Build history of the part. All positions in model axes, mm. A direction names the side the tool comes from. Give positions to 0.01 mm unless a question says otherwise; leave off trailing zeros. Order: outer loops, then holes, each group sorted by start corner. A loop starts at its lowest first (then second) coordinate and runs counter-clockwise, first axis right, second up. Notation, with made-up numbers: (-6, 5.25) - (30, 5.25) arc R24 ccw to (30, 24.25) - close; hole circle Ø8 at (39, -24). An arc over 180 degrees is marked (long way). One line per item, written item: value.
```python
from build123d import *

# Parameters (mm, degrees)
SKETCH_1_W          = 56
SKETCH_1_H          = 70
EXTRUDE_1_DEPTH     = 5
SKETCH_2_R          = 2
CUT_EXTRUDE_1_DEPTH = 5
SKETCH_5_W          = 25
SKETCH_5_H          = 28.7
EXTRUDE_3_DEPTH     = 4.5
SKETCH_6_W          = 32
SKETCH_6_H          = 40
EXTRUDE_4_DEPTH     = 15
SKETCH_9_R          = 2.15
CUT_EXTRUDE_2_DEPTH = 10
CUT_EXTRUDE_3_DEPTH = 10
CHAMFER_START       = -5
CHAMFER_1_DEPTH     = 40
CHAMFER_1_2_DEPTH   = 10
CHAMFER_START_2     = 25
CHAMFER_1_3_DEPTH   = 10
CHAMFER_START_3     = 5
CHAMFER_1_4_DEPTH   = 3
CHAMFER_2_SIZE      = 15
CHAMFER_3_SIZE      = 5


with BuildPart() as part:
    # 草图1 → 凸台-拉伸1 (new body)
    with BuildSketch(Plane.XY):
        Rectangle(SKETCH_1_W, SKETCH_1_H)
    extrude(amount=EXTRUDE_1_DEPTH)

    # 草图2 → 切除-拉伸1 (cut)
    with BuildSketch(Plane.XY.offset(5)):
        with Locations((-16, -28.4)):
            Circle(SKETCH_2_R)
        with Locations((-16, -14.4)):
            Circle(SKETCH_2_R)
    cut_extrude_1 = extrude(amount=-CUT_EXTRUDE_1_DEPTH, mode=Mode.SUBTRACT)

    # 镜向1: 切除-拉伸1 across plane
    add(cut_extrude_1.mirror(Plane(origin=(0, 0, 0), x_dir=(0, 0, 1), z_dir=(1, 0, 0))), mode=Mode.SUBTRACT)

    # 草图5 → 凸台-拉伸3 (add)
    with BuildSketch(Plane.XY.offset(5)):
        with Locations((15.5, 20.65)):
            Rectangle(SKETCH_5_W, SKETCH_5_H)
    extrude(amount=EXTRUDE_3_DEPTH)

    # 草图6 → 凸台-拉伸4 (add)
    with BuildSketch(Plane.ZY.offset(28)):
        with Locations((16, 15)):
            Rectangle(SKETCH_6_W, SKETCH_6_H)
    extrude(amount=EXTRUDE_4_DEPTH)

    # 草图9 → 切除-拉伸2 (cut)
    with BuildSketch(Plane.XY.offset(32)):
        with Locations((-35.5, 28)):
            Circle(SKETCH_9_R)
        with Locations(Location((-35.5, 2, 0), (0, 0, 180))):
            Circle(SKETCH_9_R)
    extrude(amount=-CUT_EXTRUDE_2_DEPTH, mode=Mode.SUBTRACT)

    # 草图10 → 切除-拉伸3 (cut)
    with BuildSketch(Plane.XY.offset(5)):
        with BuildLine():
            Line((-20, 5), (-20, 25))
            ThreePointArc((-20, 25), (-18, 27), (-16, 25))
            Line((-16, 25), (-16, 5))
            ThreePointArc((-16, 5), (-18, 3), (-20, 5))
        make_face()
    extrude(amount=-CUT_EXTRUDE_3_DEPTH, mode=Mode.SUBTRACT)

    # 倒角1: read off the stored shape, not the designer's step
    # 倒角1 outline → 倒角1 (add)
    with BuildSketch(Plane(origin=(0, 0, 0), x_dir=(1, 0, 0), z_dir=(0, 1, 0)).offset(CHAMFER_START)):
        Polygon((-20, -7), (-20, -5), (-28, -5), (-28, -15), align=None)
    extrude(amount=CHAMFER_1_DEPTH)

    # Chamfer 1 2 outline → Chamfer 1 2 (add)
    with BuildSketch(Plane(origin=(0, 0, 0), x_dir=(1, 0, 0), z_dir=(0, 1, 0)).offset(CHAMFER_START)):
        Polygon((-18, -5), (-20, -5), (-20, -7), align=None)
    extrude(amount=CHAMFER_1_2_DEPTH)

    # Chamfer 1 3 outline → Chamfer 1 3 (add)
    with BuildSketch(Plane(origin=(0, 0, 0), x_dir=(1, 0, 0), z_dir=(0, 1, 0)).offset(CHAMFER_START_2)):
        Polygon((-18, -5), (-20, -5), (-20, -7), align=None)
    extrude(amount=CHAMFER_1_3_DEPTH)

    # Chamfer 1 4 outline → Chamfer 1 4 (cut)
    with BuildSketch(Plane.XY.offset(CHAMFER_START_3)):
        with BuildLine():
            Line((-16, 5), (-20, 5))
            ThreePointArc((-20, 5), (-18, 3), (-16, 5))
        make_face()
        with BuildLine():
            Line((-20, 25), (-16, 25))
            ThreePointArc((-16, 25), (-18, 27), (-20, 25))
        make_face()
    extrude(amount=CHAMFER_1_4_DEPTH, mode=Mode.SUBTRACT)

    # 倒角2
    chamfer_2_edges = [part.edges().sort_by_distance(p)[0] for p in [
        (-28, -5, 2.5),
    ]]
    chamfer(chamfer_2_edges, length=CHAMFER_2_SIZE - 0.0001)  # a hair under: the kernel refuses the full size

    # 倒角3
    chamfer_3_edges = [part.edges().sort_by_distance(p)[0] for p in [
        (-30.49995, -5, 5),
    ]]
    chamfer(chamfer_3_edges, length=CHAMFER_3_SIZE)


solid = part.part
```
(1) Drill centre lines: line 1 (Y direction, x = 16, z = 3.75); line 2 (Y direction, x = 15.5, z = 1); line 3 (X direction, y = 17, z = 3). Where is each one in solid material? Low to high.
Completed:
line 1: -35 to -30.4, -26.4 to -16.4, -12.4 to 35
line 2: -35 to -30.34, -26.46 to -16.34, -12.46 to 35
line 3: -43 to -20, -16 to 28
(2) Slice it at B-B, the plane y = 23.5. Give the cut face in (x, z).
Completed:
outline: (-43, 0) - (-20, 0) - (-20, 7) - (-28, 15) - (-28, 32) - (-43, 32) - close; (-16, 0) - (28, 0) - (28, 9.5) - (3, 9.5) - (3, 5) - (-16, 5) - close
(3) Pull direction Y, two halves, no side cores. Call faces 4 (the face through (-35, 15, 32)), 5 (the face through (-31, -7, 8)), 6 (the face through (-18.643, 3.106, 2.771)): +Y half, -Y half, draft (parallel to the pull), parting line (faces both ways), or undercut.
Completed:
face 4: draft
face 5: -Y half
face 6: undercut
(4) Pin check, flat tips, straight feed: P1, Ø1.3, axis at x = 19.5, z = 8, coming from the -Y side; P2, Ø1, axis at x = -34.5, z = 14.5, coming from the -Y side; P3, Ø20, axis at x = -2, y = -17, coming from the +Z side. Stop position of each tip, or through.
Completed:
P1: y = 6.3
P2: y = -5
P3: z = 5
(5) Slice it at D-D, the plane x = -17. Give the cut face in (y, z), and give its area (3 significant figures).
Completed:
outline: (-35, 0) - (-30.13, 0) - (-30.13, 5) - (-35, 5) - close; (-26.67, 0) - (-16.13, 0) - (-16.13, 5) - (-26.67, 5) - close; (-12.67, 0) - (3.27, 0) - (3.27, 5) - (-12.67, 5) - close; (26.73, 0) - (35, 0) - (35, 5) - (26.73, 5) - close
area: 198 mm²
(6) Slice it at A-A, the plane x = 16. Give the cut face in (y, z).
Completed:
outline: (-35, 0) - (-30.4, 0) - (-30.4, 5) - (-35, 5) - close; (-26.4, 0) - (-16.4, 0) - (-16.4, 5) - (-26.4, 5) - close; (-12.4, 0) - (35, 0) - (35, 9.5) - (6.3, 9.5) - (6.3, 5) - (-12.4, 5) - close
(7) Slice it at C-C, the plane z = 24.5. Give the cut face in (x, y).
Completed:
outline: (-43, -5) - (-28, -5) - (-28, 35) - (-43, 35) - close; hole circle Ø4.3 at (-35.5, 2); hole circle Ø4.3 at (-35.5, 28)
(8) 3-axis set-ups, long thin cutter, end or side, ignore diameter. For faces 1 (the face through (-36, 28, 22)), 2 (the face through (-28, -28, 2)), 3 (the face through (-20, 15, 4)): which of +Z, -Z, +X, -X, +Y, -Y reach the whole face in a straight line?
Completed:
face 1: +Z
face 2: +Z, -Z, -X, -Y
face 3: +Z, -Z
